```python
from build123d import *

# Parameters (mm, degrees)
ESQUISSE1_W                  = 20
ESQUISSE1_H                  = 18
BOSS_EXTRU_1_DEPTH           = 6
ENL_V_MAT_EXTRU_1_DEPTH      = 28.568097504
ENL_V_MAT_EXTRU_1_DEPTH_BACK = 28.568097504
ESQUISSE4_W                  = 20.759147063
ESQUISSE4_H                  = 17.8
ENL_V_MAT_EXTRU_3_DEPTH      = 1
CONG_2_R                     = 40


with BuildPart() as part:
    # Esquisse1 → Boss.-Extru.1 (new body)
    with BuildSketch(Plane.XY):
        with Locations((10, 3)):
            Rectangle(ESQUISSE1_W, ESQUISSE1_H)
    extrude(amount=BOSS_EXTRU_1_DEPTH)

    # Esquisse2 → Enlèv. mat.-Extru.1 (cut, two sides: drawn at the far end of the back side and taken through both)
    with BuildSketch(Plane(origin=(0, 12, 0), x_dir=(1, 0, 0), z_dir=(0, 1, 0)).offset(-ENL_V_MAT_EXTRU_1_DEPTH_BACK)):
        Polygon((70.960283861, 9.63154869), (20.045630921, -0.0408989), (0, -3.849042594), (0, 0), (0, 51.825265329), (52.974270305, 140.916001049), (123.934554166, 98.72228441), align=None)
    extrude(amount=ENL_V_MAT_EXTRU_1_DEPTH + ENL_V_MAT_EXTRU_1_DEPTH_BACK, mode=Mode.SUBTRACT)

    # Esquisse4 → Enlèv. mat.-Extru.3 (cut)
    with BuildSketch(Plane(origin=(0.705746644, 0, 3.714969257), x_dir=(-0.9824291803850712, 0, 0.1866357562952965), z_dir=(-0.1866357562952965, 0, -0.9824291803850712))):
        with Locations((-9.259758994, 3)):
            Rectangle(ESQUISSE4_W, ESQUISSE4_H)
    extrude(amount=-ENL_V_MAT_EXTRU_3_DEPTH, mode=Mode.SUBTRACT)

    # Congé2
    # the kernel refuses this fillet: 40 mm, written as the material it adds along each edge
    with BuildSketch(Plane(origin=(41.830053891, 11.9, -3.079684565), x_dir=(0, -1, 0), z_dir=(-0.9824291803850712, 0, 0.1866357562952965))) as cong_2_piece_1_section:
        with BuildLine():
            CenterArc((8.888194417, -40), CONG_2_R, 90, 12.838568141)
            Line((0, -1), (0, 0))
            Line((0, 0), (8.888194417, 0))
        make_face()
    cong_2_piece_1 = extrude(amount=64.798673587, mode=Mode.PRIVATE)
    cong_2_piece_1 = split(cong_2_piece_1, bisect_by=Plane(origin=(20, 11.9, -3.079684565), z_dir=(-1, 0, 0)), keep=Keep.TOP, mode=Mode.PRIVATE)
    cong_2_piece_1 = split(cong_2_piece_1, bisect_by=Plane(origin=(0, 11.9, -3.079684565), z_dir=(1, 0, 0)), keep=Keep.TOP, mode=Mode.PRIVATE)
    add(cong_2_piece_1)
    with BuildSketch(Plane(origin=(-21.830053891, -5.9, 9.014064887), x_dir=(-0.1866357562952965, 0, -0.9824291803850712), z_dir=(0.9824291803850712, 0, -0.1866357562952965))) as cong_2_piece_2_section:
        with BuildLine():
            CenterArc((40, 8.888194417), CONG_2_R, 180, 12.838568141)
            Line((0, 8.888194417), (0, 0))
            Line((0, 0), (1, 0))
        make_face()
    cong_2_piece_2 = extrude(amount=64.798673587, mode=Mode.PRIVATE)
    cong_2_piece_2 = split(cong_2_piece_2, bisect_by=Plane(origin=(20, -5.9, 9.014064887), z_dir=(-1, 0, 0)), keep=Keep.TOP, mode=Mode.PRIVATE)
    cong_2_piece_2 = split(cong_2_piece_2, bisect_by=Plane(origin=(0, -5.9, 9.014064887), z_dir=(1, 0, 0)), keep=Keep.TOP, mode=Mode.PRIVATE)
    add(cong_2_piece_2)


solid = part.part
```
Verification items for the finished model (mm, model axes). A direction names the side the tool comes from. Coordinates: 2 decimals unless noted, no trailing zeros. Write each loop counter-clockwise with the first axis right and the second up, starting at its lowest first coordinate (ties: lowest second). Pieces come first, ordered by that corner, then holes. Notation, with made-up numbers: (43, 52.5) - (63, 52.5) arc R15 ccw to (63, 59.5) - close; hole circle Ø9 at (-20.75, -8.5). An arc over 180 degrees is marked (long way). Write item = value, one per line.
Q1. Cross-section at B-B (y = 2). Enter the section's corners in (x, z).
Answer:
outline = (0, 4.85) - (20, 1.06) - (20, 6) - (0, 6) - close
Q2. Mould release check, pull along Y, two halves, no side actions. Record for faces 3 (the face through (10.189, 7.422, 2.683)), 4 (the face through (12, 12, 4)), 5 (the face through (20, 3, 3)): released by +Y, released by -Y, zero draft, split by the parting line, or undercut.
Answer:
face_3 = undercut
face_4 = released by +Y
face_5 = zero draft
Q3. Cross-section at A-A (y = -3.25). Enter the section's corners in (x, z).
Answer:
outline = (0, 4.37) - (20, 0.57) - (20, 6) - (0, 6) - close
Q4. Material ranges on L1, parallel to Z at x = 3, y = 9.5; L2, parallel to Z at x = 9, y = 4.5, recorded low to high. Write a range as from..to.
Answer:
L1 = 3.76..6
L2 = 3.13..6
Q5. Access from +Z, -Z, +X, -X, +Y, -Y to the whole of each face (thin tool, end or side, straight path). Record for faces 1 (the face through (9.907, -1.422, 2.737)), 2 (the face through (10, 3, 6)).
Answer:
face_1 = -Z, -X
face_2 = +Z, +X, -X, +Y, -Y
